Read the model definition and answer for the solid it produces. Units are mm, in the model's axes. Face numbers are marked on the shaded views. A direction names the side the tool comes from. Round coordinates to 2 decimals unless told otherwise and drop trailing zeros. Loops run counter-clockwise (first coordinate to the right, second up) from the corner with the lowest first, then second, coordinate; pieces in that order, holes last. Notation, with made-up numbers: (-10.75, -22) - (6.25, -22) arc R24 cw to (6.25, 11) - close; hole circle Ø8 at (21, 13). An arc over 180 degrees is marked (long way). Answer as CSV lines item,"result".
Autodesk Inventor part; units mm, degrees
ref_plane "YZ Plane" through (0, 0, 0) normal (1, 0, 0) x (0, 1, 0)
ref_plane "XZ Plane" through (0, 0, 0) normal (0, 1, 0) x (-1, 0, 0)
ref_plane "XY Plane" through (0, 0, 0) normal (0, 0, 1) x (1, 0, 0)
sketch "Sketch1" plane through (0, 0, 0) normal (0, 1, 0) x (-1, 0, 0)
  line L0 (3.175, 0) -> (47.625, 0)
  line L1 (50.8, -3.175) -> (50.8, -73.025)
  line L2 (47.625, -76.2) -> (3.175, -76.2)
  line L3 (0, -73.025) -> (0, -3.175)
  arc A0 (50.8, -3.175) -> (47.625, 0) centre (47.625, -3.175) ccw
  arc A1 (3.175, 0) -> (0, -3.175) centre (3.175, -3.175) ccw
  arc A2 (0, -73.025) -> (3.175, -76.2) centre (3.175, -73.025) ccw
  arc A3 (47.625, -76.2) -> (50.8, -73.025) centre (47.625, -73.025) ccw
  point P0 (0, 0)
  point P1 (50.8, -76.2)
  point P2 (50.8, 0)
  point P3 (0, -76.2)
  dimension "d0" = 50.8
  dimension "d1" = 76.2
  dimension "d4" = 3.175
extrude "Extrusion1" add sketch "Sketch1" along normal blind 12.7
sketch "Sketch2" plane through (0, 12.7, 0) normal (0, 1, 0) x (1, 0, 0)
  line L0 (0, 0) -> (-6.35, 0) construction
  line L1 (-6.35, 0) -> (-6.35, 6.35) construction
  line L2 (-6.35, 6.35) -> (0, 6.35) construction
  line L3 (0, 6.35) -> (0, 0) construction
  circle A0 centre (-6.35, 6.35) radius 3.175
  line L4 (0, 3.175) -> (0, 73.025) construction
  line L5 (0, 38.1) -> (-50.8802, 38.1) construction
  line L6 (-50.8802, 38.1) -> (-25.4, 76.2) construction
  line L7 (-3.175, 76.2) -> (-47.625, 76.2) construction
  line L8 (-25.4, 76.2) -> (-25.4, 0) construction
  line L9 (-47.625, 0) -> (-3.175, 0) construction
  circle A1 centre (-6.35, 69.85) radius 3.175
  circle A2 centre (-44.45, 6.35) radius 3.175
  circle A3 centre (-44.45, 69.85) radius 3.175
  dimension "d5" = 6.35
  dimension "d6" = 6.35
  dimension "d7" = 6.35
extrude "Extrusion2" cut sketch "Sketch2" against normal through all
sketch "Sketch3" plane through (0, 12.7, 0) normal (0, 1, 0) x (1, 0, 0)
  line L0 (0, 0) -> (-12.7, 0) construction
  line L1 (0, 0) -> (12.7, 0) construction
  line L2 (-47.625, 0) -> (-3.175, 0) construction
  line L3 (-25.4, 0) -> (-25.4, 76.2) construction
  line L4 (-3.175, 76.2) -> (-47.625, 76.2) construction
  line L5 (-50.8, 0) -> (-38.1, 0) construction
  line L6 (-38.1, 0) -> (-13.2855, 0)
  line L7 (-13.2855, 0) -> (-13.2855, 76.2)
  line L8 (-13.2855, 76.2) -> (-38.1, 76.2)
  line L9 (-38.1, 76.2) -> (-38.1, 0)
  dimension "d14" = 12.7
  dimension "d15" = 180
extrude "Extrusion3" add sketch "Sketch3" along normal blind 38.1
sketch "Sketch4" plane through (0, 0, 0) normal (0, -1, 0) x (1, 0, 0)
  line L0 (0, 0) -> (-12.7, 0) construction
  line L1 (-12.7, 0) -> (-12.7, -12.7) construction
  line L2 (-12.7, -12.7) -> (0, -12.7) construction
  line L3 (0, -12.7) -> (0, 0) construction
  line L4 (-50.8, -76.2) -> (-38.1, -76.2) construction
  line L5 (-38.1, -76.2) -> (-38.1, -63.5) construction
  line L6 (-38.1, -63.5) -> (-50.8, -63.5) construction
  line L7 (-50.8, -63.5) -> (-50.8, -76.2) construction
  line L8 (-12.7, -12.7) -> (-38.1, -12.7)
  line L9 (-38.1, -12.7) -> (-38.1, -63.5)
  line L10 (-38.1, -63.5) -> (-12.7, -63.5)
  line L11 (-12.7, -63.5) -> (-12.7, -12.7)
  dimension "d18" = 12.7
  dimension "d19" = 12.7
  dimension "d20" = 12.7
  dimension "d21" = 12.7
extrude "Extrusion4" cut sketch "Sketch4" against normal blind 6.35
properties part number "Near Gantry Bracket"
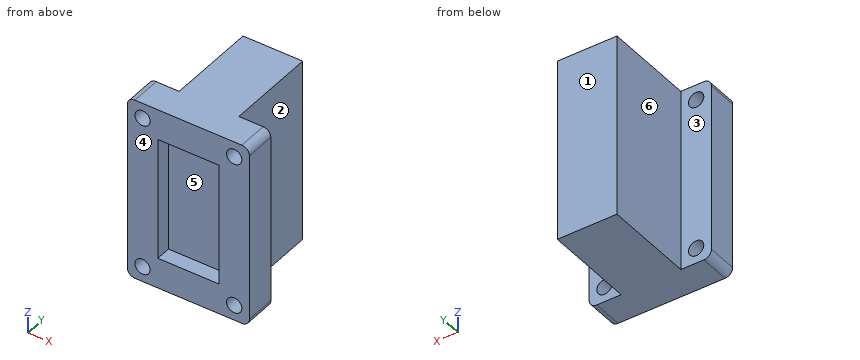
1) Find the intervals of material crossed by line 1 (X direction, y = 4, z = -6.35) (3 decimals); line 2 (Z direction, x = -44, y = 9); line 3 (X direction, y = 5.5, z = -58), in increasing order.
Entries:
line 1,"x = -50.8 to -47.625, -41.275 to -9.525, -3.175 to 0"
line 2,"z = -76.2 to -72.99, -66.71 to -9.49, -3.21 to 0"
line 3,"x = -50.8 to -38.1, -12.7 to 0"
2) A cutting plane is placed at A-A, the plane z = -6.35. Determine the outline of the cut face in (x, y) (1 decimal).
Entries:
outline,"(-50.8, 0) - (-47.6, 0) - (-47.6, 12.7) - (-50.8, 12.7) - close; (-41.3, 0) - (-9.5, 0) - (-9.5, 12.7) - (-13.3, 12.7) - (-13.3, 50.8) - (-38.1, 50.8) - (-38.1, 12.7) - (-41.3, 12.7) - close; (-3.2, 0) - (0, 0) - (0, 12.7) - (-3.2, 12.7) - close"
3) A cutting plane is placed at B-B, the plane x = -44.45. Determine the outline of the cut face in (y, z) (3 decimals), plus the area to 3 significant figures.
Entries:
outline,"(0, -76.2) - (12.7, -76.2) - (12.7, -73.025) - (0, -73.025) - close; (0, -66.675) - (12.7, -66.675) - (12.7, -9.525) - (0, -9.525) - close; (0, -3.175) - (12.7, -3.175) - (12.7, 0) - (0, 0) - close"
area,"806 mm^2"
4) Each of these flat-tipped pins is pushed along its axis until it touches: P1, Ø6, axis at y = 28.5, z = -30.5, coming from the -X side; P2, Ø6.5, axis at x = -42, z = -46, coming from the +Y side; P3, Ø11.5, axis at y = 33, z = -36, coming from the +X side. Where does it stop, or does it pass through?
Entries:
P1,"stops at x = -38.1"
P2,"stops at y = 12.7"
P3,"stops at x = -13.29"
5) A cutting plane is placed at D-D, the plane y = 42. Determine the outline of the cut face in (x, z).
Entries:
outline,"(-38.1, -76.2) - (-13.29, -76.2) - (-13.29, 0) - (-38.1, 0) - close"
6) The mould has two halves that part along X. Classify the marked faces 4, 5 and 6: pulls with the +X half, pulls with the -X half, needs draft (parallel to the pull), parting line crosses it, or undercut.
Entries:
face 4,"needs draft"
face 5,"undercut"
face 6,"pulls with the -X half"
7) A cutting plane is placed at C-C, the plane z = -58. Determine the outline of the cut face in (x, y).
Entries:
outline,"(-50.8, 0) - (-38.1, 0) - (-38.1, 6.35) - (-12.7, 6.35) - (-12.7, 0) - (0, 0) - (0, 12.7) - (-13.29, 12.7) - (-13.29, 50.8) - (-38.1, 50.8) - (-38.1, 12.7) - (-50.8, 12.7) - close"
8) A tool of negligible diameter and unlimited length cuts with its end or side. For the marked faces 1, 2 and 3, from which of +Z, -Z, +X, -X, +Y, -Y can it reach the whole face along a straight path? Write none if from no direction.
Entries:
face 1,"+Z, -Z, +X, -X, +Y"
face 2,"+Z, -Z, +X, +Y"
face 3,"+Z, -Z, -X, +Y"
